Read the model definition and answer for the solid it produces. Units are mm, in the model's axes. Face numbers are marked on the shaded views. A direction names the side the tool comes from. Give positions to 0.01 mm unless a question says otherwise; leave off trailing zeros. Write each loop counter-clockwise with the first axis right and the second up, starting at its lowest first coordinate (ties: lowest second). Pieces come first, ordered by that corner, then holes. Notation, with made-up numbers: M 32,-19 L 40,-19 A22 cw 40,11 Z; hole C -17,50.25 d2. An arc over 180 degrees is marked long. Use a Markdown table: item, result. Add a question column.
Item 1: A cutting plane is placed at C-C on z = -2.5. Determine the outline of the cut face in (x, y), then the cut area to 3 significant figures.
Item 2: Consider probe 1 along X at (y, z) = (-3, 0.25); probe 2 along X at (y, z) = (0.5, 1.25); probe 3 along X at (y, z) = (4.25, 4.75). Determine where each line is inside the solid, lowest interval first. Write a range as [from, to].
Item 3: A cutting plane is placed at B-B on y = -4. Determine the outline of the cut face in (x, z), then the cut area to 3 significant figures.
Item 4: For the marked faces 1 and 2, determine the directions among +Z, -Z, +X, -X, +Y, -Y from which every point of the face is accessible in a straight line to the end or side of a thin tool.
Item 5: Given P1, Ø3, axis at x = -48.5, y = -1, coming from the +Z side, flat-ended and moving along its own axis, determine where the tip first touches the part or whether it passes through.
Item 6: The mould has two halves that part along Z. Classify the marked faces 3, 4, 5 and 6: pulls with the +Z half, pulls with the -Z half, needs draft (parallel to the pull), parting line crosses it, or undercut.
Item 7: A cutting plane is placed at A-A on x = 0. Determine the outline of the cut face in (y, z).
from build123d import *

# Parameters (mm, degrees)
SKETCH_1_R      = 4
EXTRUDE_1_DEPTH = 5


with BuildPart() as part:
    # 草圖1 → 填料-伸長1 (new body, symmetric)
    with BuildSketch(Plane(origin=(0, 0, 0), x_dir=(1, 0, 0), z_dir=(0, 1, 0))):
        Polygon((-55, -5), (-55, 0), (-45, 0), (-45, -5), (6, -5), (6, 5), (-57, 5), (-57, -5), align=None)
        Circle(SKETCH_1_R, mode=Mode.SUBTRACT)
    extrude(amount=EXTRUDE_1_DEPTH, both=True)


solid = part.part
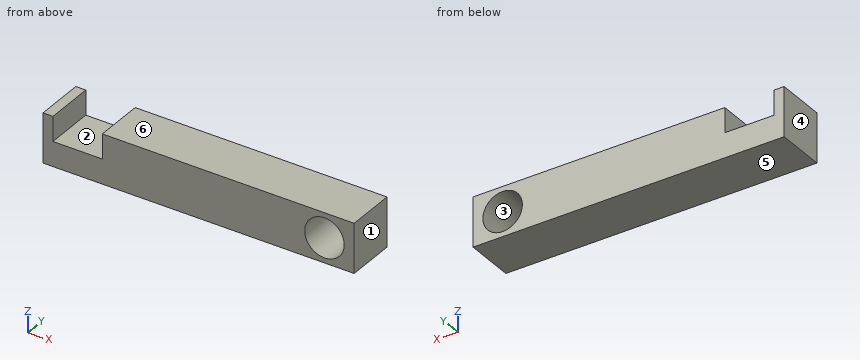
Filled in:
| question | item | result |
|---|---|---|
| 1 | outline | M -57,-5 L -3.12,-5 L -3.12,5 L -57,5 Z; M 3.12,-5 L 6,-5 L 6,5 L 3.12,5 Z |
| 1 | area | 568 mm² |
| 2 | probe 1 | [-57, -55], [-45, -3.99], [3.99, 6] |
| 2 | probe 2 | [-57, -55], [-45, -3.8], [3.8, 6] |
| 2 | probe 3 | [-57, -55], [-45, 6] |
| 3 | outline | M -57,-5 L 6,-5 L 6,5 L -45,5 L -45,0 L -55,0 L -55,5 L -57,5 Z; hole C 0,0 d8 |
| 3 | area | 530 mm² |
| 4 | face 1 | +Z, -Z, +X, +Y, -Y |
| 4 | face 2 | +Z, +Y, -Y |
| 5 | P1 | z = 0 |
| 6 | face 3 | undercut |
| 6 | face 4 | needs draft |
| 6 | face 5 | pulls with the -Z half |
| 6 | face 6 | pulls with the +Z half |
| 7 | outline | M -5,-5 L 5,-5 L 5,-4 L -5,-4 Z; M -5,4 L 5,4 L 5,5 L -5,5 Z |
